from build123d import *

# Parameters (mm, degrees)
SKETCH1_R           = 3.9116
BOSS_EXTRUDE1_DEPTH = 31.75
SKETCH2_R           = 4.699
BOSS_EXTRUDE2_DEPTH = 17.272
CUT_EXTRUDE1_START  = -1.5748
SKETCH3_R           = 4.699
SKETCH3_R_2         = 4.572
CUT_EXTRUDE1_DEPTH  = 1.5748
SKETCH6_R           = 4.7625
BOSS_EXTRUDE4_DEPTH = 12.7
SKETCH7_R           = 4.7625
SKETCH7_R_2         = 3.9751
CUT_EXTRUDE2_DEPTH  = 2.286
SKETCH8_R           = 6.35
BOSS_EXTRUDE5_DEPTH = 31.9532
CHAMFER1_SIZE       = 0.7874
CHAMFER2_SIZE       = 0.381


with BuildPart() as part:
    # Sketch1 → Boss-Extrude1 (new, symmetric)
    with BuildSketch(Plane(origin=(0, 0, 0), x_dir=(0, 0, -1), z_dir=(1, 0, 0))):
        Circle(SKETCH1_R)
    extrude(amount=BOSS_EXTRUDE1_DEPTH, both=True)

    # Sketch2 → Boss-Extrude2 (add)
    with BuildSketch(Plane.ZY.offset(31.75)):
        Circle(SKETCH2_R)
    extrude(amount=-BOSS_EXTRUDE2_DEPTH)

    # Sketch3 → Cut-Extrude1 (cut)
    with BuildSketch(Plane(origin=(-14.478, 0, 0), x_dir=(0, 0, -1), z_dir=(1, 0, 0)).offset(CUT_EXTRUDE1_START)):
        with Locations(Location((0, 0, 0), (0, 0, 180))):
            Circle(SKETCH3_R)
        Circle(SKETCH3_R_2, mode=Mode.SUBTRACT)
    extrude(amount=CUT_EXTRUDE1_DEPTH, mode=Mode.SUBTRACT)

    # Sketch6 → Boss-Extrude4 (add)
    with BuildSketch(Plane(origin=(31.75, 0, 0), x_dir=(0, 0, -1), z_dir=(1, 0, 0))):
        Circle(SKETCH6_R)
    extrude(amount=-BOSS_EXTRUDE4_DEPTH)

    # Sketch7 → Cut-Extrude2 (cut)
    with BuildSketch(Plane(origin=(31.75, 0, 0), x_dir=(0, 0, -1), z_dir=(1, 0, 0))):
        Circle(SKETCH7_R)
        Circle(SKETCH7_R_2, mode=Mode.SUBTRACT)
    extrude(amount=-CUT_EXTRUDE2_DEPTH, mode=Mode.SUBTRACT)

    # Sketch8 → Boss-Extrude5 (add)
    with BuildSketch(Plane(origin=(-14.478, 0, 0), x_dir=(0, 0, -1), z_dir=(1, 0, 0))):
        Circle(SKETCH8_R)
    extrude(amount=BOSS_EXTRUDE5_DEPTH)

    # Chamfer1
    chamfer1_edges = [part.edges().sort_by_distance(p)[0] for p in [
        (-14.478, 0, 6.35),
        (-31.75, 0, -4.699),
    ]]
    chamfer(chamfer1_edges, length=CHAMFER1_SIZE)

    # Chamfer2
    chamfer2_edges = [part.edges().sort_by_distance(p)[0] for p in [
        (31.75, 0, 3.9751),
        (17.4752, 0, 6.35),
    ]]
    chamfer(chamfer2_edges, length=CHAMFER2_SIZE)


solid = part.part
The model under review builds one solid part; all positions refer to its coordinate system, in mm. A direction names the side the tool comes from. Give positions to 0.01 mm unless a question says otherwise; leave off trailing zeros. Order: outer loops, then holes, each group sorted by start corner. A loop starts at its lowest first (then second) coordinate and runs counter-clockwise, first axis right, second up. Notation, with made-up numbers: M 64,-2 L 120,-2 A23 cw 120,24 Z; hole C -33.5,-10.5 d7. An arc over 180 degrees is marked long. Answer in a Markdown table with one row per item. Add a question column.
1. To check wall thickness, follow line 1 along X through (y, z) = (-3.75, -2.75); line 2 along X through (y, z) = (-1, 4.5); line 3 along X through (y, z) = (-3.25, 3.75). State the ranges of each line that lie inside material, in increasing order.
2. Mouldability with a two-part tool opening along X and no side actions: class faces 5 (the flat face through (31.75, 0, 0)), 6 (the cylindrical face through (1.49, -6.2, 1.38)), 7 (the cylindrical face through (18.274, 1.175, -3.731)) as released by +X, released by -X, zero draft, split by the parting line, or undercut.
3. Machinability: for faces 1 (the flat face through (-31.75, 0, 0)), 2 (the flat face through (-14.478, -5, 1)), 3 (the cylindrical face through (-23.61, 4.66, -0.61)), 4 (the cylindrical face through (24.33, -2.9, 3.78)), which of the approach directions +Z, -Z, +X, -X, +Y, -Y give a long, thin tool a straight path to every point of the face, cutting with its end or side? Answer none if there is none.
4. For pin 1 Ø1.5 at (x, z) = (23, -5) entering from +Y; pin 2 Ø2 at (x, z) = (-1.5, 4.5) entering from +Y; pin 3 Ø4 at (x, z) = (15.5, 1.5) entering from -Y; pin 4 Ø4 at (x, z) = (-2.5, 3.5) entering from -Y, all flat-tipped, find the tip position at first contact; note any pin that passes through.
5. Add section C-C on x = -9.5. State the section outline as (y, z) points.
The answers:
| question | item | result |
|---|---|---|
| 1 | line 1 | -31.01 to -16.05, -14.48 to 17.48, 19.05 to 29.46 |
| 1 | line 2 | -31.05 to -16.05, -14.48 to 17.48, 19.05 to 29.46 |
| 1 | line 3 | -14.48 to 17.48 |
| 2 | face 5 | released by +X |
| 2 | face 6 | zero draft |
| 2 | face 7 | undercut |
| 3 | face 1 | +Z, -Z, -X, +Y, -Y |
| 3 | face 2 | none |
| 3 | face 3 | -X |
| 3 | face 4 | +X |
| 4 | pin 1 | y = 2.15 |
| 4 | pin 2 | y = 5.3 |
| 4 | pin 3 | y = -6.35 |
| 4 | pin 4 | y = -6.17 |
| 5 | outline | C 0,0 d12.7 |
